Here's how the part is built. I have some questions about the finished solid (model axes, mm). Coordinates: 2 decimals unless noted, no trailing zeros. Order: outer loops, then holes, each group sorted by start corner. A loop starts at its lowest first (then second) coordinate and runs counter-clockwise, first axis right, second up. Notation, with made-up numbers: (80, 48.5) - (133, 48.5) arc R4 ccw to (133, 52.5) - close; hole circle Ø9 at (80.25, 48.25). An arc over 180 degrees is marked (long way). Answer as CSV lines item,"result". Start each with the question number.
Q1. Suppose I cut it at A-A (z = 377.5). Please give me the cut outline in (x, y), then the cut area to 3 significant figures.
Q2. Suppose I cut it at B-B (y = -4.75). Count the separate pieces of the cut face and the enclosed holes in it, then the cut area to 3 significant figures.
Q3. For pin 1 Ø8 at (y, z) = (-6.5, 225) entering from -X; pin 2 Ø1.8 at (x, z) = (-1.5, 165.5) entering from -Y; pin 3 Ø12 at (x, z) = (-7.5, 190) entering from +Y; pin 4 Ø6 at (x, z) = (0.5, 778) entering from -Y, each with a flat end and sliding along its axis, tell me the tip position at first contact or that it passes through.
Q4. I need wall thicknesses on line 1 (X direction, y = -4.5, z = 465); line 2 (X direction, y = 1.5, z = 776); line 3 (Y direction, x = 1.75, z = 710). Which ranges of each line are inside material? Lowest first, please.
from build123d import *

# Parameters (mm, degrees)
SKETCH1_R           = 10
BOSS_EXTRUDE1_DEPTH = 1000
CHAMFER1_SIZE       = 1
SKETCH2_R           = 3
CUT_EXTRUDE1_DEPTH  = 10
LPATTERN1_COUNT     = 7
LPATTERN1_PITCH     = 150


with BuildPart() as part:
    # Sketch1 → Boss-Extrude1 (new body)
    with BuildSketch(Plane.XY):
        Circle(SKETCH1_R)
    extrude(amount=BOSS_EXTRUDE1_DEPTH)

    # Chamfer1
    chamfer1_edges = [part.edges().sort_by_distance(p)[0] for p in [
        (-10, 0, 0),
        (-10, 0, 1000),
    ]]
    chamfer(chamfer1_edges, length=CHAMFER1_SIZE)

    # Sketch2 → Cut-Extrude1 (cut)
    with BuildSketch(Plane(origin=(0, 0, 0), x_dir=(1, 0, 0), z_dir=(0, 1, 0))):
        with Locations((0, -15)):
            Circle(SKETCH2_R)
    cut_extrude1 = extrude(amount=-CUT_EXTRUDE1_DEPTH, mode=Mode.SUBTRACT)

    # LPattern1: Cut-Extrude1 ×7
    with Locations(*[(0, 0, i * LPATTERN1_PITCH) for i in range(1, LPATTERN1_COUNT)]):
        add(cut_extrude1, mode=Mode.SUBTRACT)


solid = part.part
Here are the results:
1,outline,"circle Ø20 at (0, 0)"
1,area,"314 mm²"
2,separate pieces,"1"
2,enclosed holes,"7"
2,area,"17,400 mm²"
3,pin 1,"stops at x = -9.68"
3,pin 2,"stops at y = 0"
3,pin 3,"stops at y = 9.89"
3,pin 4,"stops at y = -10"
4,line 1,"x = -8.93 to -3, 3 to 8.93"
4,line 2,"x = -9.89 to 9.89"
4,line 3,"y = -9.85 to 9.85"
